Autodesk Inventor part; units mm, degrees
ref_plane "YZ Plane" through (0, 0, 0) normal (1, 0, 0) x (0, 1, 0)
ref_plane "XZ Plane" through (0, 0, 0) normal (0, 1, 0) x (-1, 0, 0)
ref_plane "XY Plane" through (0, 0, 0) normal (0, 0, 1) x (1, 0, 0)
sketch "Szkic1" plane through (0, 0, 0) normal (0, 1, 0) x (-1, 0, 0)
  line L0 (-22.5, -45) -> (22.5, -45)
  line L1 (22.5, -45) -> (22.5, 45)
  line L2 (22.5, 45) -> (-22.5, 45)
  line L3 (-22.5, 45) -> (-22.5, -45)
  line L4 (-22.5, -45) -> (22.5, 45) construction
  line L5 (22.5, -45) -> (-22.5, 45) construction
  point P0 (0, 0)
  dimension "d0" = 45
  dimension "d1" = 90
extrude "Wyciągnięcie proste1" add sketch "Szkic1" along normal blind 2
sketch "Szkic2" plane through (0, 2, 0) normal (0, 1, 0) x (1, 0, 0)
  line L0 (11.5, 3.5) -> (18.5, 3.5)
  line L1 (18.5, 3.5) -> (18.5, 35.5)
  line L2 (18.5, 35.5) -> (-20.5, 35.5)
  line L3 (-20.5, 35.5) -> (-20.5, -35.5)
  line L4 (-20.5, -35.5) -> (18.5, -35.5)
  line L5 (18.5, -35.5) -> (18.5, -26.5)
  line L6 (18.5, -26.5) -> (11.5, -26.5)
  line L7 (11.5, -26.5) -> (11.5, 3.5)
  circle A0 centre (6, 0) radius 1.5
  circle A1 centre (14, 31.5) radius 1.5
  circle A2 centre (-16, -31.5) radius 1.5
  circle A3 centre (-16, 31.5) radius 1.5
  circle A4 centre (14, -31.5) radius 1.5
  circle A5 centre (-16, 0) radius 1.5
  point P0 (0, 0)
hole "Otwór1" at (14, 2, -31.5) at (6, 2, 0) at (14, 2, 31.5) at (-16, 2, 31.5) at (-16, 2, 0) at (-16, 2, -31.5) direction (0, -1, 0) diameter 3.5 end through all
properties part number "blacha pionowa"
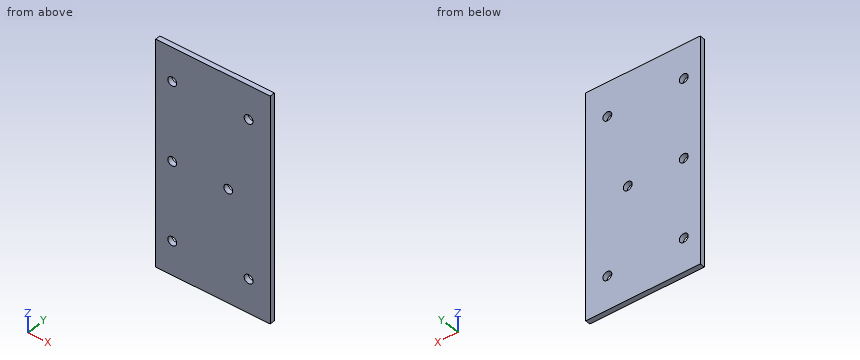
Input: part model. Units: mm. Frame: model coordinates. Give positions to 0.01 mm unless a question says otherwise; leave off trailing zeros. Write each loop counter-clockwise with the first axis right and the second up, starting at its lowest first coordinate (ties: lowest second). Pieces come first, ordered by that corner, then holes. Notation, with made-up numbers: (-31.75, 34) - (-11.75, 34) arc R10 ccw to (-11.75, 48) - close; hole circle Ø2 at (22.5, -29). An arc over 180 degrees is marked (long way). Write item = value, one per line. Start each with the question number.
1. Ray query, L1, parallel to X at y = 1.15, z = 31.5; L2, parallel to X at y = 1.6, z = 0; L3, parallel to Z at x = -16, y = 0.8. Return the intervals inside material, ascending.
2. Section query C-C, the plane x = 14. Output: boundary loops of the cut face in (y, z).
3. First-contact query: pin 1 Ø5.5 at (x, z) = (-16, 0) entering from +Y; pin 2 Ø2 at (x, z) = (-16, 31.5) entering from +Y. Flat tips, straight axial feed; report the tip coordinate or a pass-through.
4. Section query A-A, the plane x = 6. Output: boundary loops of the cut face in (y, z).
5. Section query B-B, the plane z = 31.5. Output: boundary loops of the cut face in (x, y), then the cut area to 3 significant figures.
Check sheet entries:
q1.L1 = -22.5 to -17.75, -14.25 to 12.25, 15.75 to 22.5
q1.L2 = -22.5 to -17.75, -14.25 to 4.25, 7.75 to 22.5
q1.L3 = -45 to -33.25, -29.75 to -1.75, 1.75 to 29.75, 33.25 to 45
q2.outline = (0, -45) - (2, -45) - (2, -33.25) - (0, -33.25) - close; (0, -29.75) - (2, -29.75) - (2, 29.75) - (0, 29.75) - close; (0, 33.25) - (2, 33.25) - (2, 45) - (0, 45) - close
q3.pin_1 = 2
q3.pin_2 = through
q4.outline = (0, -45) - (2, -45) - (2, -1.75) - (0, -1.75) - close; (0, 1.75) - (2, 1.75) - (2, 45) - (0, 45) - close
q5.outline = (-22.5, 0) - (-17.75, 0) - (-17.75, 2) - (-22.5, 2) - close; (-14.25, 0) - (12.25, 0) - (12.25, 2) - (-14.25, 2) - close; (15.75, 0) - (22.5, 0) - (22.5, 2) - (15.75, 2) - close
q5.area = 76.0 mm2
